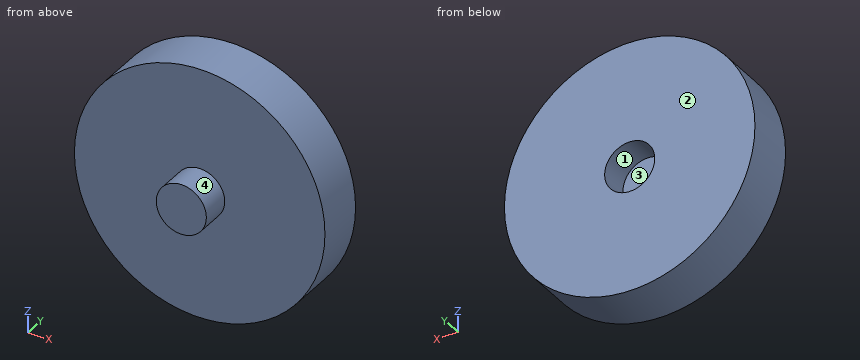
Autodesk Inventor part; units mm, degrees
ref_plane "YZ Plane" through (0, 0, 0) normal (1, 0, 0) x (0, 1, 0)
ref_plane "XZ Plane" through (0, 0, 0) normal (0, 1, 0) x (-1, 0, 0)
ref_plane "XY Plane" through (0, 0, 0) normal (0, 0, 1) x (1, 0, 0)
sketch "スケッチ1" plane through (0, 0, 0) normal (0, 1, 0) x (-1, 0, 0)
  circle A0 centre (0, 0) radius 12.5
  dimension "d0" = 25
extrude "押し出し1" add sketch "スケッチ1" along normal blind 5
sketch "スケッチ2" plane through (0, 5, 0) normal (0, 1, 0) x (1, 0, 0)
  circle A0 centre (0, 0) radius 12.5
  circle A1 centre (0, 0) radius 2.5
  dimension "d3" = 5
extrude "押し出し2" cut sketch "スケッチ2" against normal blind 3 contours A1
sketch "スケッチ3" plane through (0, 0, 0) normal (0, -1, 0) x (1, 0, 0)
  circle A0 centre (0, 0) radius 12.5
  circle A1 centre (0, 0) radius 2.5
  dimension "d6" = 5
extrude "押し出し3" add sketch "スケッチ3" along normal blind 3 contours A1
properties part number "知能ロボコンシリンダ延長5mm"
Part model, mm, in its own coordinate system. Face numbers are marked on the shaded views. Coordinates: 2 decimals unless noted, no trailing zeros. Order: outer loops, then holes, each group sorted by start corner. A loop starts at its lowest first (then second) coordinate and runs counter-clockwise, first axis right, second up. Notation, with made-up numbers: (58.25, 55.25) - (102.25, 55.25) arc R26 ccw to (102.25, 89.25) - close; hole circle Ø8 at (-9, 11.25). An arc over 180 degrees is marked (long way). Return JSON: item names as keys, results as strings. Group by question number.
Item 1: Pin check, flat tips, straight feed: pin 1 (1.5 mm diameter, centred on x = -0.5, z = 0.5, fed in from +Y); pin 2 (2 mm diameter, centred on x = 9, z = -4, fed in from -Y); pin 3 (4 mm diameter, centred on y = -1.5, z = -3, fed in from -X). Stop position of each tip, or through.
Item 2: Pull direction X, two halves, no side cores. Call the marked faces 1, 2, 3 and 4: pulls with the +X half, pulls with the -X half, needs draft (parallel to the pull), parting line crosses it, or undercut.
Item 3: Cut at D-D (y = 0.75). List the corners of the cut face in (x, z).
Item 4: Drill centre lines: probe 1 along Z at (x, y) = (0, 2.7); probe 2 along Y at (x, z) = (-4, -7); probe 3 along Z at (x, y) = (-2, 0.5). Where is each one in solid material? Low to high. Write a range as from..to.
Item 5: Cut at B-B (z = 0). List the corners of the cut face in (x, y).
Item 6: Cut at C-C (y = 3.5). List the corners of the cut face in (x, z), plus the area to 3 significant figures.
Item 7: Cut at A-A (x = 0). List the corners of the cut face in (y, z), plus the area to 3 significant figures.
Check values:
{
 "1": {"pin 1": "stops at y = 2", "pin 2": "stops at y = 0", "pin 3": "stops at x = -12.39"},
 "2": {"face 1": "undercut", "face 2": "needs draft", "face 3": "undercut", "face 4": "parting line crosses it"},
 "3": {"outline": "circle Ø25 at (0, 0)"},
 "4": {"probe 1": "z = -12.5..-2.5, 2.5..12.5", "probe 2": "y = 0..5", "probe 3": "z = -12.34..12.34"},
 "5": {"outline": "(-12.5, 0) - (-2.5, 0) - (-2.5, -3) - (2.5, -3) - (2.5, 0) - (12.5, 0) - (12.5, 5) - (2.5, 5) - (2.5, 2) - (-2.5, 2) - (-2.5, 5) - (-12.5, 5) - close"},
 "6": {"outline": "circle Ø25 at (0, 0); hole circle Ø5 at (0, 0)", "area": "471 mm2"},
 "7": {"outline": "(-3, -2.5) - (0, -2.5) - (0, -12.5) - (5, -12.5) - (5, -2.5) - (2, -2.5) - (2, 2.5) - (5, 2.5) - (5, 12.5) - (0, 12.5) - (0, 2.5) - (-3, 2.5) - close", "area": "125 mm2"}
}
